from build123d import *

# Parameters (mm, degrees)
SKETCH1_W                = 60
SKETCH1_H                = 60
BOSS_EXTRUDE1_DEPTH      = 10
SKETCH2_W                = 40
SKETCH2_H                = 35
CUT_EXTRUDE1_DEPTH       = 40
BOSS_EXTRUDE8_DEPTH      = 20
BOSS_EXTRUDE8_DEPTH_BACK = 10
BOSS_EXTRUDE9_DEPTH      = 10
SKETCH3_R                = 6.35
CUT_EXTRUDE2_DEPTH       = 40


with BuildPart() as part:
    # Sketch1 → Boss-Extrude1 (new body)
    with BuildSketch(Plane.XY):
        Rectangle(SKETCH1_W, SKETCH1_H)
    extrude(amount=BOSS_EXTRUDE1_DEPTH)

    # Sketch2 → Cut-Extrude1 (cut)
    with BuildSketch(Plane.XY.offset(10)):
        with Locations((-10, 12.5)):
            Rectangle(SKETCH2_W, SKETCH2_H)
    extrude(amount=-CUT_EXTRUDE1_DEPTH, mode=Mode.SUBTRACT)

    # Sketch6 → Boss-Extrude8 (add, two sides: drawn at the far end of the back side and taken through both)
    with BuildSketch(Plane(origin=(0, 0, 0), x_dir=(-1, 0, 0), z_dir=(0, 0, -1)).offset(-BOSS_EXTRUDE8_DEPTH_BACK)):
        Polygon((-10, 30), (-5, 30), (-5, -5), (30, -5), (30, -30), (-10, -30), align=None)
    extrude(amount=BOSS_EXTRUDE8_DEPTH + BOSS_EXTRUDE8_DEPTH_BACK)

    # Sketch7 → Boss-Extrude9 (add)
    with BuildSketch(Plane(origin=(0, 0, -20), x_dir=(-1, 0, 0), z_dir=(0, 0, -1))):
        Polygon((-30, 30), (-5, 30), (-5, -5), (30, -5), (30, -30), (-30, -30), align=None)
    extrude(amount=BOSS_EXTRUDE9_DEPTH)

    # Sketch3 → Cut-Extrude2 (cut, symmetric)
    with BuildSketch(Plane.XY.offset(10)):
        with Locations(Location((20, -20, 0), (0, 0, 180))):
            Circle(SKETCH3_R)
        with Locations(Location((20, 20, 0), (0, 0, 180))):
            Circle(SKETCH3_R)
    extrude(amount=CUT_EXTRUDE2_DEPTH, both=True, mode=Mode.SUBTRACT)


solid = part.part
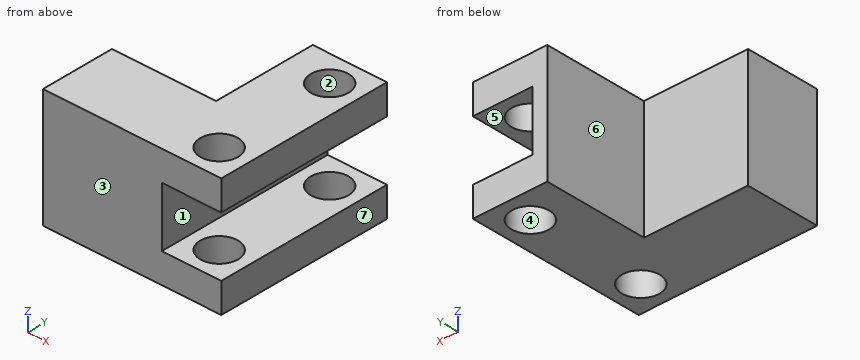
Geometry check sheet. Reference: the model listing, model coordinates, mm. Face numbers are marked on the shaded views. A direction names the side the tool comes from. Give positions to 0.01 mm unless a question says otherwise; leave off trailing zeros. Loops run counter-clockwise (first coordinate to the right, second up) from the corner with the lowest first, then second, coordinate; pieces in that order, holes last. Notation, with made-up numbers: (38, 4.5) -> (46, 4.5) arc R25 cw to (46, 28.5) -> close; hole circle Ø1 at (-30, 46.5). An arc over 180 degrees is marked (long way). Answer in a Markdown table with one row per item. Add a question column.
1) Cross-section at A-A on y = -20. Record the boundary of the cut face in (x, z).
2) Cross-section at B-B on z = -25. Record the boundary of the cut face in (x, y).
3) Set-up check for the marked faces 5, 6 and 7: record each of +Z, -Z, +X, -X, +Y, -Y from which the full face is reachable in a straight line by a thin tool's end or side.
4) Material ranges on probe 1 along Y at (x, z) = (20, 7.5); probe 2 along Z at (x, y) = (16.5, -1); probe 3 along X at (y, z) = (20, 7.25), recorded low to high. Write a range as from..to.
5) Gauge pin test, flat ends, axial feed: P1, Ø4, axis at y = 16.5, z = -12.5, coming from the +X side; P2, Ø7.5, axis at x = 20, y = 20, coming from the +Z side. Record the tip position at first contact, or that the pin passes through.
6) Draft check along Y on the marked faces 1, 2, 3 and 4. Enter one of: pulls with the +Y half, pulls with the -Y half, needs draft (parallel to the pull), parting line crosses it, or undercut.
7) Cross-section at C-C on x = 20. Record the boundary of the cut face in (y, z).
8) Cross-section at D-D on y = -10.5. Record the boundary of the cut face in (x, z), and give its area (3 significant figures).
Outcome:
| question | item | result |
|---|---|---|
| 1 | outline | (-30, -30) -> (13.65, -30) -> (13.65, -20) -> (10, -20) -> (10, 0) -> (13.65, 0) -> (13.65, 10) -> (-30, 10) -> close; (26.35, -30) -> (30, -30) -> (30, -20) -> (26.35, -20) -> close; (26.35, 0) -> (30, 0) -> (30, 10) -> (26.35, 10) -> close |
| 2 | outline | (-30, -30) -> (30, -30) -> (30, 30) -> (5, 30) -> (5, -5) -> (-30, -5) -> close; hole circle Ø12.7 at (20, -20); hole circle Ø12.7 at (20, 20) |
| 3 | face 5 | +X, +Y, -Y |
| 3 | face 6 | +Z, -Z, -X, +Y |
| 3 | face 7 | +Z, -Z, +X, +Y, -Y |
| 4 | probe 1 | y = -30..-26.35, -13.65..13.65, 26.35..30 |
| 4 | probe 2 | z = -30..-20, 0..10 |
| 4 | probe 3 | x = 5..13.65, 26.35..30 |
| 5 | P1 | stops at x = 10 |
| 5 | P2 | passes through |
| 6 | face 1 | needs draft |
| 6 | face 2 | undercut |
| 6 | face 3 | pulls with the -Y half |
| 6 | face 4 | undercut |
| 7 | outline | (-30, -30) -> (-26.35, -30) -> (-26.35, -20) -> (-30, -20) -> close; (-30, 0) -> (-26.35, 0) -> (-26.35, 10) -> (-30, 10) -> close; (-13.65, -30) -> (13.65, -30) -> (13.65, -20) -> (-13.65, -20) -> close; (-13.65, 0) -> (13.65, 0) -> (13.65, 10) -> (-13.65, 10) -> close; (26.35, -30) -> (30, -30) -> (30, -20) -> (26.35, -20) -> close; (26.35, 0) -> (30, 0) -> (30, 10) -> (26.35, 10) -> close |
| 8 | outline | (-30, -30) -> (30, -30) -> (30, -20) -> (10, -20) -> (10, 0) -> (30, 0) -> (30, 10) -> (-30, 10) -> close |
| 8 | area | 2,000 mm^2 |
